Autodesk Inventor part; units mm, degrees
ref_plane "YZ Plane" through (0, 0, 0) normal (1, 0, 0) x (0, 1, 0)
ref_plane "XZ Plane" through (0, 0, 0) normal (0, 1, 0) x (-1, 0, 0)
ref_plane "XY Plane" through (0, 0, 0) normal (0, 0, 1) x (1, 0, 0)
sketch "Sketch1" plane through (0, 0, 0) normal (0, 0, 1) x (1, 0, 0)
  line L0 (0, 0) -> (508, 0)
  line L1 (508, 0) -> (508, 508)
  line L2 (508, 508) -> (0, 508)
  line L3 (0, 508) -> (0, 0)
  line L4 (0, 254) -> (508, 254) construction
  line L5 (254, 508) -> (254, 0) construction
  line L6 (25.4, 482.6) -> (482.6, 482.6) construction
  line L7 (482.6, 482.6) -> (482.6, 25.4) construction
  line L8 (482.6, 25.4) -> (25.4, 25.4) construction
  line L9 (25.4, 25.4) -> (25.4, 482.6) construction
  circle A0 centre (6.35, 501.65) radius 2.4892
  circle A1 centre (501.65, 501.65) radius 2.4892
  circle A2 centre (501.65, 6.35) radius 2.4892
  circle A3 centre (6.35, 6.35) radius 2.4892
  line L10 (254, 254) -> (25.4, 254) construction
  circle A4 centre (6.35, 406.4) radius 2.4892
  circle A5 centre (6.35, 393.7) radius 2.4892
  circle A6 centre (19.05, 406.4) radius 2.4892
  circle A7 centre (19.05, 393.7) radius 2.4892
  circle A8 centre (6.35, 101.6) radius 2.4892
  circle A9 centre (6.35, 114.3) radius 2.4892
  circle A10 centre (19.05, 101.6) radius 2.4892
  circle A11 centre (19.05, 114.3) radius 2.4892
  line L11 (0, 292.1) -> (19.05, 292.1) construction
  line L12 (19.05, 292.1) -> (19.05, 215.9) construction
  line L13 (19.05, 215.9) -> (0, 215.9) construction
  line L14 (0, 215.9) -> (0, 292.1) construction
  circle A12 centre (12.7, 279.4) radius 2.4892
  circle A13 centre (12.7, 228.6) radius 2.4892
  circle A14 centre (12.7, 254) radius 2.4892
  dimension "d5" = 508
  dimension "d6" = 508
  dimension "d12" = 25.4
  dimension "d67" = 4.9784
  dimension "d69" = 6.35
  dimension "d70" = 6.35
  dimension "d106" = 4.9784
  dimension "d109" = 12.7
  dimension "d112" = 12.7
  dimension "d115" = 6.35
  dimension "d116" = 101.6
  dimension "d117" = 19.05
  dimension "d118" = 76.2
  dimension "d119" = 4.9784
  dimension "d120" = 12.7
  dimension "d121" = 6.35
  dimension "d123" = 6.35
extrude "Extrusion1" add sketch "Sketch1" along normal blind 0.7937
sketch "Sketch3" plane through (0, 0, 0) normal (0, 0, -1) x (-1, 0, 0)
  line L0 (-508, 508) -> (0, 508)
  line L1 (-508, 0) -> (-508, 508)
  circle A0 centre (-444.5, 444.5) radius 38.1
  dimension "d26" = 76.2
  dimension "d27" = 63.5
  dimension "d28" = 63.5
extrude "Extrusion3" cut sketch "Sketch3" against normal blind 1.5875
pattern_linear "Rectangular Pattern1" count 4 spacing 127 along (-1, 0, 0) count 4 spacing 127 along (0, -1, 0) of "Extrusion3"
sketch "Sketch4" plane through (0, 0, 0.7937) normal (0, 0, 1) x (1, 0, 0)
  circle A0 centre (12.7, 254) radius 2.4892
  line L0 (508, 0) -> (508, 508)
  line L1 (0, 508) -> (0, 0)
  line L2 (63.5, 266.7) -> (50.8, 266.7) construction
  line L3 (50.8, 266.7) -> (50.8, 241.3) construction
  line L4 (50.8, 241.3) -> (63.5, 241.3) construction
  line L5 (63.5, 241.3) -> (63.5, 266.7) construction
  line L6 (0, 254) -> (508, 254) construction
  circle A1 centre (57.15, 260.35) radius 2.4892
  circle A2 centre (57.15, 247.65) radius 2.4892
  dimension "d124" = 25.4
  dimension "d125" = 12.7
  dimension "d126" = 4.9784
  dimension "d127" = 6.35
  dimension "d130" = 50.8
  dimension "d131" = 6.35
extrude "Extrusion4" cut sketch "Sketch4" against normal blind 25.4 contours A1 | A2
equation "\"BendRadius\" = Thickness"
equation "\"BendReliefWidth\" = Thickness"
equation "\"BendReliefDepth\" = 0.5 * Thickness"
equation "\"CornerReliefSize\" = 4 * Thickness"
equation "\"MinimumRemnant\" = 2 * Thickness"
equation "\"TransitionRadius\" = BendRadius"
equation "\"JacobiRadiusSize\" = Thickness"
equation "\"GapSize\" = Thickness"
properties part number "Plastic Funnel PIece" material "Polycarbonate, Clear"
The listing builds one solid part. Answer for the finished solid, in the listing's coordinates (mm). Coordinates: 2 decimals unless noted, no trailing zeros. Loops run counter-clockwise (first coordinate to the right, second up) from the corner with the lowest first, then second, coordinate; pieces in that order, holes last. Notation, with made-up numbers: (52.25, 21.5) - (94.25, 21.5) arc R14 ccw to (94.25, 45.5) - close; hole circle Ø3 at (48.5, -15.5). An arc over 180 degrees is marked (long way). Use a Markdown table: item, result. Add a question column.
1) Find the intervals of material crossed by line 1 (Y direction, x = 444.5, z = 0.2); line 2 (Y direction, x = 19.05, z = 0.6); line 3 (X direction, y = 426.5, z = 0.4), in increasing order.
2) The mould has two halves that part along X. Classify faces 1 (the flat face through (250, 258, 0.794)), 2 (the cylindrical face through (198.759, 153.306, 0.391)): released by +X, released by -X, zero draft, split by the parting line, or undercut.
3) The part is cut by section C-C, the plane z = 0.6. State how many separate pieces and enclosed holes the cut face has, and give its area (3 significant figures).
4) The part is cut by section A-A, the plane y = 190.5. Give the vertices of the cut face in (x, z).
5) Given pin 1 (8 mm diameter, centred on x = 12.7, y = 254, fed in from -Z); pin 2 (4 mm diameter, centred on x = 19.05, y = 101.6, fed in from +Z), each flat-ended and moving along its own axis, determine where each tip first touches the part or whether it passes through.
Here are the results:
| question | item | result |
|---|---|---|
| 1 | line 1 | y = 0 to 25.4, 101.6 to 152.4, 228.6 to 279.4, 355.6 to 406.4, 482.6 to 508 |
| 1 | line 2 | y = 0 to 99.11, 104.09 to 111.81, 116.79 to 391.21, 396.19 to 403.91, 408.89 to 508 |
| 1 | line 3 | x = 0 to 29.92, 97.08 to 156.92, 224.08 to 283.92, 351.08 to 410.92, 478.08 to 508 |
| 2 | face 1 | zero draft |
| 2 | face 2 | undercut |
| 3 | separate pieces | 1 |
| 3 | enclosed holes | 33 |
| 3 | area | 185,000 mm^2 |
| 4 | outline | (0, 0) - (25.4, 0) - (25.4, 0.79) - (0, 0.79) - close; (101.6, 0) - (152.4, 0) - (152.4, 0.79) - (101.6, 0.79) - close; (228.6, 0) - (279.4, 0) - (279.4, 0.79) - (228.6, 0.79) - close; (355.6, 0) - (406.4, 0) - (406.4, 0.79) - (355.6, 0.79) - close; (482.6, 0) - (508, 0) - (508, 0.79) - (482.6, 0.79) - close |
| 5 | pin 1 | stops at z = 0 |
| 5 | pin 2 | passes through |
